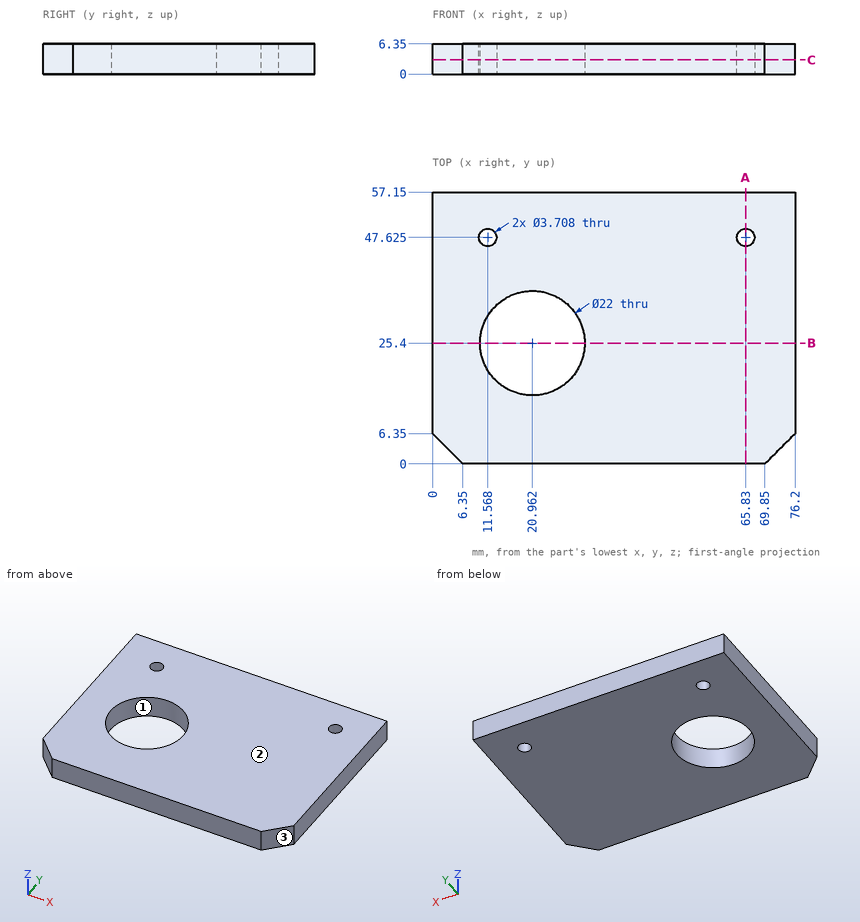
Here's the drawing with two shaded views (mm, measured from the low corner). I have some questions. Coordinates: 2 decimals unless noted, no trailing zeros. Loops run counter-clockwise (first coordinate to the right, second up) from the corner with the lowest first, then second, coordinate; pieces in that order, holes last. Notation, with made-up numbers: (77.5, -27.75) -> (87.5, -27.75) arc R20 cw to (87.5, -17.75) -> close; hole circle Ø11 at (56, -25). An arc over 180 degrees is marked (long way). Put each result on its own line as item: value. Start each with the question number.
Q1. If I drill on line 1 (X direction, y = 25.5, z = 0.5); line 2 (Y direction, x = 65.83, z = 3); line 3 (X direction, y = 29, z = 5.25), over which ranges is the centre line in solid material (lowest first)? Write a range as [from, to].
Q2. Thinking about a two-plate mould opening in X: for the marked faces 1, 2 and 3, which applies, pulls with the +X half, pulls with the -X half, needs draft (parallel to the pull), parting line crosses it, or undercut?
Q3. I want a section at B-B (y = 25.4). Write out the boundary of the cut face in (x, z).
Q4. I want a section at A-A (x = 65.83). Write out the boundary of the cut face in (y, z), plus the area to 3 significant figures.
Q5. I want a section at C-C (z = 3). Count the separate pieces of the cut face and the enclosed holes in it, plus the area to 3 significant figures.
Taken from the geometry:
1. line 1: x = [0, 9.96], [31.96, 76.2]
1. line 2: y = [0, 45.77], [49.48, 57.15]
1. line 3: x = [0, 10.57], [31.36, 76.2]
2. face 1: undercut
2. face 2: needs draft
2. face 3: pulls with the +X half
3. outline: (0, 0) -> (9.96, 0) -> (9.96, 6.35) -> (0, 6.35) -> close; (31.96, 0) -> (76.2, 0) -> (76.2, 6.35) -> (31.96, 6.35) -> close
4. outline: (0, 0) -> (45.77, 0) -> (45.77, 6.35) -> (0, 6.35) -> close; (49.48, 0) -> (57.15, 0) -> (57.15, 6.35) -> (49.48, 6.35) -> close
4. area: 339 mm2
5. separate pieces: 1
5. enclosed holes: 3
5. area: 3,910 mm2
